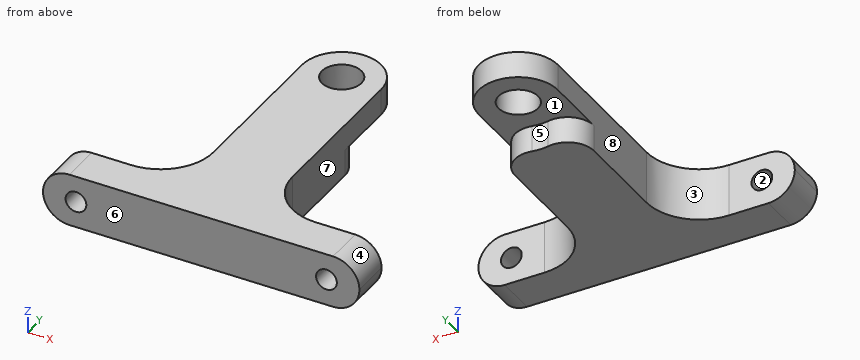
```python
from build123d import *

# Parameters (mm, degrees)
SKETCH2_R           = 9.525
SKETCH2_R_2         = 4.7625
BOSS_EXTRUDE1_DEPTH = 12.7
FILLET1_R           = 12.7
SKETCH3_R           = 2.5
CUT_EXTRUDE1_DEPTH  = 35.56
FILLET2_R           = 6.35
SKETCH4_R           = 4.7625
CUT_EXTRUDE2_DEPTH  = 6.35
FILLET3_START       = -1
FILLET3_DEPTH       = 7.35


with BuildPart() as part:
    # Sketch2 → Boss-Extrude1 (new body)
    # profile 1 of 2: a face of its own
    with BuildSketch(Plane.XY):
        with BuildLine():
            ThreePointArc((9.525, 0), (0, -9.525), (-9.525, 0))
            Line((-9.525, 0), (-9.525, -50.8))
            Line((-9.525, -50.8), (-38.1, -50.8))
            Line((-38.1, -50.8), (-38.1, -60.325))
            Line((-38.1, -60.325), (38.1, -60.325))
            Line((38.1, -60.325), (38.1, -50.8))
            Line((38.1, -50.8), (9.525, -50.8))
            Line((9.525, -50.8), (9.525, 0))
        make_face()
    # profile 2 of 2: a face of its own
    with BuildSketch(Plane.XY):
        Circle(SKETCH2_R)
        Circle(SKETCH2_R_2, mode=Mode.SUBTRACT)
    extrude(amount=BOSS_EXTRUDE1_DEPTH)

    # Fillet1
    fillet1_edges = [part.edges().sort_by_distance(p)[0] for p in [
        (9.525, -50.8, 6.35),
        (-9.525, -50.8, 6.35),
    ]]
    fillet(fillet1_edges, radius=FILLET1_R)

    # Sketch3 → Cut-Extrude1 (cut)
    with BuildSketch(Plane(origin=(0, -50.8, 0), x_dir=(1, 0, 0), z_dir=(0, 1, 0))):
        with Locations(Location((30.1625, -6.35, 0), (0, 0, 180))):
            Circle(SKETCH3_R)
        with Locations(Location((-30.1625, -6.35, 0), (0, 0, 180))):
            Circle(SKETCH3_R)
    extrude(amount=-CUT_EXTRUDE1_DEPTH, mode=Mode.SUBTRACT)

    # Fillet2
    fillet2_edges = [part.edges().sort_by_distance(p)[0] for p in [
        (38.1, -55.5625, 0),
        (38.1, -55.5625, 12.7),
        (-38.1, -55.5625, 0),
        (-38.1, -55.5625, 12.7),
    ]]
    fillet(fillet2_edges, radius=FILLET2_R - 0.0001)  # a hair under: the kernel refuses the full size

    # Sketch4 → Cut-Extrude2 (cut)
    with BuildSketch(Plane(origin=(0, 0, 0), x_dir=(-1, 0, 0), z_dir=(0, 0, -1))):
        with BuildLine():
            ThreePointArc((-9.525, 0), (0, -9.525), (9.525, 0))
            ThreePointArc((9.525, 0), (0, 9.525), (-9.525, 0))
        make_face()
        with Locations(Location((0, 0, 0), (0, 0, 180))):
            Circle(SKETCH4_R, mode=Mode.SUBTRACT)
    extrude(amount=-CUT_EXTRUDE2_DEPTH, mode=Mode.SUBTRACT)

    # Fillet3: read off the stored shape, not the designer's step
    # Fillet3 outline → Fillet3 (cut)
    with BuildSketch(Plane.XY.offset(FILLET3_START)):
        with BuildLine():
            Line((-9.525, 0), (-9.525, -15.554259867))
            ThreePointArc((-9.525, -15.554259867), (-7.191092628, -10.635571017), (-1.905, -9.33255592))
            ThreePointArc((-1.905, -9.33255592), (-7.378033275, -6.024138943), (-9.525, 0))
        make_face()
        with BuildLine():
            ThreePointArc((9.525, 0), (7.378033275, -6.024138943), (1.905, -9.33255592))
            ThreePointArc((1.905, -9.33255592), (7.191092628, -10.635571017), (9.525, -15.554259867))
            Line((9.525, -15.554259867), (9.525, 0))
        make_face()
    extrude(amount=FILLET3_DEPTH, mode=Mode.SUBTRACT)


solid = part.part
```
The listing builds one solid part. Answer for the finished solid, in the listing's coordinates (mm). Face numbers are marked on the shaded views. A direction names the side the tool comes from. Give positions to 0.01 mm unless a question says otherwise; leave off trailing zeros. Order: outer loops, then holes, each group sorted by start corner. A loop starts at its lowest first (then second) coordinate and runs counter-clockwise, first axis right, second up. Notation, with made-up numbers: (59, 54) -> (95, 54) arc R14 cw to (95, 59) -> close; hole circle Ø3 at (60, -37.5). An arc over 180 degrees is marked (long way). One line per item, written item: value.
1) Find section C-C, the plane y = -27. Determine the outline of the cut face in (x, z) (3 decimals), plus the area to 3 significant figures.
Reported:
outline: (-9.525, 0) -> (9.525, 0) -> (9.525, 12.7) -> (-9.525, 12.7) -> close
area: 242 mm^2
2) Flat-ended cylindrical pins translate along their axes: P1, Ø21, axis at x = 4.5, y = -3, coming from the -Z side; P2, Ø4.5, axis at x = -30.16, z = 6.35, coming from the -Y side; P3, Ø4, axis at y = -25, z = 7, coming from the -X side (3 decimals); P4, Ø3, axis at y = -44, z = 3, coming from the -X side. Find the tip coordinate at first contact, or state that the pin passes through.
Reported:
P1: stops at z = 0
P2: passes through
P3: stops at x = -9.525
P4: stops at x = -11.9
3) Determine the mould class of the marked faces 1, 2 and 3 for opening direction Z: pulls with the +Z half, pulls with the -Z half, needs draft (parallel to the pull), parting line crosses it, or undercut.
Reported:
face 1: pulls with the -Z half
face 2: undercut
face 3: needs draft
4) Find section D-D, the plane z = 2. Determine the outline of the cut face in (x, y) (3 decimals).
Reported:
outline: (-36.376, -60.325) -> (36.376, -60.325) -> (36.376, -50.8) -> (22.225, -50.8) arc R12.7 cw to (9.525, -38.1) -> (9.525, -15.554) arc R6.35 ccw to (1.905, -9.333) arc R9.525 cw to (-1.905, -9.333) arc R6.35 ccw to (-9.525, -15.554) -> (-9.525, -38.1) arc R12.7 cw to (-22.225, -50.8) -> (-36.376, -50.8) -> close
5) Find the intervals of material crossed by line 1 (Y direction, x = 0, z = 11) (1 decimal); line 2 (X direction, y = -14.5, z = 12.25) (3 decimals); line 3 (Y direction, x = 25, z = 0.75) (3 decimals), in increasing order.
Reported:
line 1: y = -60.3 to -4.8, 4.8 to 9.5
line 2: x = -9.525 to 9.525
line 3: y = -60.325 to -50.8
6) A tool of negligible diameter and unlimited length cuts with its end or side. For the marked faces 4, 5, 6, 7 and 8, from which of +Z, -Z, +X, -X, +Y, -Y can it reach the whole face along a straight path? Write none if from no direction.
Reported:
face 4: +Z, +X, +Y, -Y
face 5: -Z, +Y
face 6: +Z, -Z, +X, -X, -Y
face 7: +Z, -Z, +X, +Y
face 8: +Z, -Z, -X, +Y
7) Find section A-A, the plane z = 7.25. Count the separate pieces of the cut face and the enclosed holes in it, plus the area to 3 significant figures.
Reported:
separate pieces: 3
enclosed holes: 1
area: 1,740 mm^2
